from build123d import *

# Parameters (mm, degrees)
SKETCH002_W          = 278
SKETCH002_H          = 278
PAD002_DEPTH         = 6
POCKET_DEPTH         = 0.001
POCKET_DEPTH_BACK    = 6.001
SKETCH004_R          = 2
POCKET001_DEPTH      = 6.001
POCKET001_DEPTH_BACK = 0.001
FILLET_R             = 3


with BuildPart() as part:
    # Sketch002 → Pad002 (new body)
    with BuildSketch(Plane.XY):
        Rectangle(SKETCH002_W, SKETCH002_H)
    extrude(amount=PAD002_DEPTH)

    # Sketch003 → Pocket (cut, two sides)
    with BuildSketch(Plane.XY) as pocket_sk:
        Polygon((-79, 125), (79, 125), (79, 102), (102, 79), (125, 79), (125, -79), (102, -79), (79, -102), (79, -125), (-79, -125), (-79, -102), (-102, -79), (-125, -79), (-125, 79), (-102, 79), (-79, 102), align=None)
    extrude(amount=-POCKET_DEPTH, mode=Mode.SUBTRACT)
    extrude(pocket_sk.sketch, amount=POCKET_DEPTH_BACK, mode=Mode.SUBTRACT)

    # Sketch004 (on Face5 of Pad002) → Pocket001 (cut, two sides)
    with BuildSketch(Plane(origin=(0, 0, 0), x_dir=(1, 0, 0), z_dir=(0, 0, -1))) as pocket001_sk:
        with Locations((-125, 125)):
            Circle(SKETCH004_R)
        with Locations((125, 125)):
            Circle(SKETCH004_R)
        with Locations((125, -125)):
            Circle(SKETCH004_R)
        with Locations((-125, -125)):
            Circle(SKETCH004_R)
    extrude(amount=-POCKET001_DEPTH, mode=Mode.SUBTRACT)
    extrude(pocket001_sk.sketch, amount=POCKET001_DEPTH_BACK, mode=Mode.SUBTRACT)

    # Fillet
    fillet_edges = [part.edges().sort_by_distance(p)[0] for p in [
        (-90.5, -90.5, 6),
        (-90.5, 90.5, 6),
        (90.5, 90.5, 6),
        (90.5, -90.5, 6),
    ]]
    fillet(fillet_edges, radius=FILLET_R)


solid = part.part
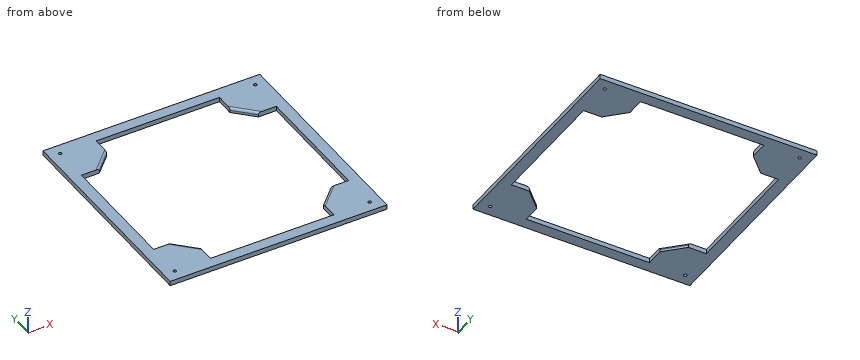
Work out the finished part from the listing and answer in its coordinate system (mm). Give positions to 0.01 mm unless a question says otherwise; leave off trailing zeros. Order: outer loops, then holes, each group sorted by start corner. A loop starts at its lowest first (then second) coordinate and runs counter-clockwise, first axis right, second up. Notation, with made-up numbers: (27.5, 50) - (57.5, 50) arc R32 cw to (57.5, 85) - close; hole circle Ø2 at (27.25, 77.5). An arc over 180 degrees is marked (long way). Answer as CSV lines item,"result". Start each with the question number.
Q1. Given pin 1 Ø5 at (x, y) = (125, -125) entering from +Z, flat-ended and moving along its own axis, determine where the tip first touches the part or whether it passes through.
Q2. The part is cut by section A-A (y = -3). Write down the section's boundary in (x, z).
Q3. The part is cut by section C-C (z = 1.75). Write down the section's boundary in (x, y).
Q4. Find the intervals of material crossed by L1, parallel to X at y = 7.5, z = 3.5; L2, parallel to Y at x = 109, z = 1, in increasing order. Write a range as [from, to].
Check result:
1,pin 1,"stops at z = 6"
2,outline,"(-139, 0) - (-125, 0) - (-125, 6) - (-139, 6) - close; (125, 0) - (139, 0) - (139, 6) - (125, 6) - close"
3,outline,"(-139, -139) - (139, -139) - (139, 139) - (-139, 139) - close; hole circle Ø4 at (-125, -125); hole circle Ø4 at (-125, 125); hole (-125, -79) - (-102, -79) - (-79, -102) - (-79, -125) - (79, -125) - (79, -102) - (102, -79) - (125, -79) - (125, 79) - (102, 79) - (79, 102) - (79, 125) - (-79, 125) - (-79, 102) - (-102, 79) - (-125, 79) - close; hole circle Ø4 at (125, -125); hole circle Ø4 at (125, 125)"
4,L1,"x = [-139, -125], [125, 139]"
4,L2,"y = [-139, -79], [79, 139]"
